Study the drawing (mm; zero at the part's minimum x, y, z) and answer. A direction names the side the tool comes from. Coordinates: 2 decimals unless noted, no trailing zeros. Loops run counter-clockwise (first coordinate to the right, second up) from the corner with the lowest first, then second, coordinate; pieces in that order, holes last. Notation, with made-up numbers: (8, 10) -> (34, 10) arc R16 ccw to (34, 26) -> close; hole circle Ø11 at (72, 12.5). An arc over 180 degrees is marked (long way). Answer as CSV lines item,"result".
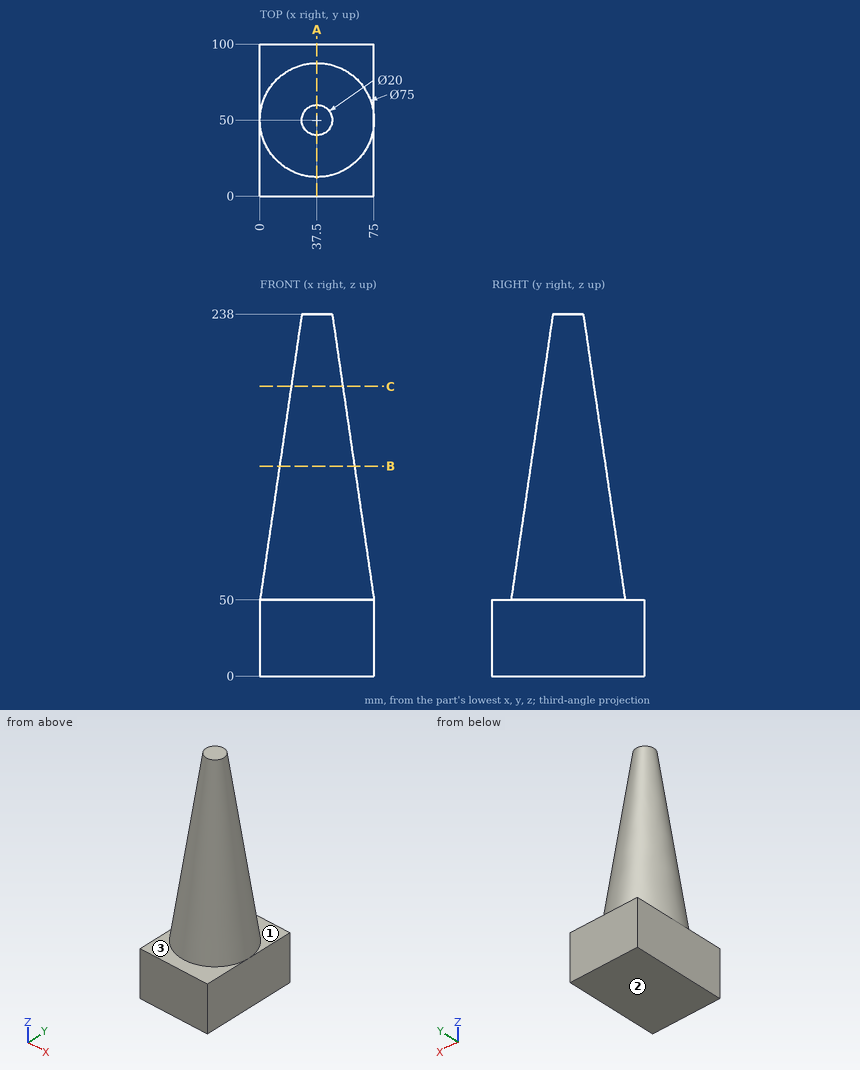
Q1. For the marked faces 1, 2 and 3, determine the directions among +Z, -Z, +X, -X, +Y, -Y from which every point of the face is accessible in a straight line to the end or side of a thin tool.
Results:
face 1,"+Z, +Y"
face 2,"-Z, +X, -X, +Y, -Y"
face 3,"+Z, -Y"
Q2. A cutting plane is placed at B-B, the plane z = 138. Write down the section's boundary in (x, y), and give its area (3 significant figures).
Results:
outline,"circle Ø49.26 at (37.5, 50)"
area,"1,910 mm²"
Q3. Given pin 1 Ø10 at (y, z) = (50.5, 116) entering from -X; pin 2 Ø6 at (x, z) = (29.5, 185) entering from +Y; pin 3 Ø5 at (x, z) = (17, 100) entering from -Y, each flat-ended and moving along its own axis, determine where each tip first touches the part or whether it passes through.
Results:
pin 1,"stops at x = 8.92"
pin 2,"stops at y = 67.14"
pin 3,"stops at y = 25.71"
Q4. A cutting plane is placed at C-C, the plane z = 190.5. Write down the section's boundary in (x, y).
Results:
outline,"circle Ø33.9 at (37.5, 50)"
Q5. Find the intervals of material crossed by probe 1 along Z at (x, y) = (45.5, 8); probe 2 along Y at (x, z) = (36, 175); probe 3 along Y at (x, z) = (42, 143.5), in increasing order. Write a range as [from, to].
Results:
probe 1,"z = [0, 50]"
probe 2,"y = [30.84, 69.16]"
probe 3,"y = [26.61, 73.39]"
Q6. A cutting plane is placed at A-A, the plane x = 37.5. Write down the section's boundary in (y, z), and give its area (3 significant figures).
Results:
outline,"(0, 0) -> (100, 0) -> (100, 50) -> (87.5, 50) -> (60, 238) -> (40, 238) -> (12.5, 50) -> (0, 50) -> close"
area,"13,900 mm²"
